```python
from build123d import *

# Parameters (mm, degrees)
SKETCH1_W           = 130
SKETCH1_H           = 120
BOSS_EXTRUDE1_DEPTH = 40
CUT_EXTRUDE1_DEPTH  = 40
CUT_EXTRUDE2_DEPTH  = 10
SKETCH4_R           = 10
CUT_EXTRUDE4_DEPTH  = 159
CUT_EXTRUDE5_DEPTH  = 20
SKETCH7_R           = 10
CUT_EXTRUDE6_DEPTH  = 20
CUT_EXTRUDE7_DEPTH  = 10


with BuildPart() as part:
    # Sketch1 → Boss-Extrude1 (new body)
    with BuildSketch(Plane.XY):
        with Locations((65, 60)):
            Rectangle(SKETCH1_W, SKETCH1_H)
    extrude(amount=BOSS_EXTRUDE1_DEPTH)

    # Sketch2 → Cut-Extrude1 (cut)
    with BuildSketch(Plane.XY.offset(40)):
        with BuildLine():
            Line((0, 70), (20, 70))
            ThreePointArc((20, 70), (30, 60), (20, 50))
            Line((20, 50), (0, 50))
            Line((0, 50), (0, 70))
        make_face()
    extrude(amount=-CUT_EXTRUDE1_DEPTH, mode=Mode.SUBTRACT)

    # Sketch3 → Cut-Extrude2 (cut)
    with BuildSketch(Plane.XY.offset(40)):
        with BuildLine():
            Line((20, 90), (0, 90))
            Line((0, 90), (0, 70))
            Line((0, 70), (20, 70))
            ThreePointArc((20, 70), (30, 60), (20, 50))
            Line((20, 50), (0, 50))
            Line((0, 50), (0, 30))
            Line((0, 30), (20, 30))
            ThreePointArc((20, 30), (50, 60), (20, 90))
        make_face()
    extrude(amount=-CUT_EXTRUDE2_DEPTH, mode=Mode.SUBTRACT)

    # Sketch4 → Cut-Extrude4 (cut)
    with BuildSketch(Plane.XY.offset(40)):
        with Locations((70, 60)):
            Circle(SKETCH4_R)
    extrude(amount=-CUT_EXTRUDE4_DEPTH, mode=Mode.SUBTRACT)

    # Sketch6 → Cut-Extrude5 (cut)
    with BuildSketch(Plane.XY.offset(30)):
        with BuildLine():
            Line((0, 90), (20, 90))
            ThreePointArc((20, 90), (50, 60), (20, 30))
            Line((20, 30), (0, 30))
            Line((0, 30), (0, 50))
            Line((0, 50), (20, 50))
            ThreePointArc((20, 50), (30, 60), (20, 70))
            Line((20, 70), (0, 70))
            Line((0, 70), (0, 90))
        make_face()
    extrude(amount=-CUT_EXTRUDE5_DEPTH, mode=Mode.SUBTRACT)

    # Sketch7 → Cut-Extrude6 (cut)
    with BuildSketch(Plane.XY.offset(40)):
        with BuildLine():
            Line((0, 120), (0, 90))
            Line((0, 90), (20, 90))
            ThreePointArc((20, 90), (50, 60), (20, 30))
            Line((20, 30), (0, 30))
            Line((0, 30), (0, 0))
            Line((0, 0), (70, 0))
            Line((70, 0), (70, 20))
            ThreePointArc((70, 20), (110, 60), (70, 100))
            Line((70, 100), (70, 120))
            Line((70, 120), (0, 120))
        make_face()
        with Locations((70, 60)):
            Circle(SKETCH7_R, mode=Mode.SUBTRACT)
    extrude(amount=-CUT_EXTRUDE6_DEPTH, mode=Mode.SUBTRACT)

    # Sketch8 → Cut-Extrude7 (cut)
    with BuildSketch(Plane.XY.offset(40)):
        with BuildLine():
            Line((96.457513111, 90), (130, 90))
            Line((130, 90), (130, 30))
            Line((130, 30), (96.457513111, 30))
            ThreePointArc((96.457513111, 30), (110, 60), (96.457513111, 90))
        make_face()
    extrude(amount=-CUT_EXTRUDE7_DEPTH, mode=Mode.SUBTRACT)


solid = part.part
```
Can you work these out from the model? Positions are in its coordinate system, mm. A direction names the side the tool comes from. Round coordinates to 2 decimals unless told otherwise and drop trailing zeros. Loops run counter-clockwise (first coordinate to the right, second up) from the corner with the lowest first, then second, coordinate; pieces in that order, holes last.
Item 1: Which directions (+Z, -Z, +X, -X, +Y, -Y) give clear straight access to the entire face, cutting with the end or side of a thin tool? Please do faces 1 (the flat face through (113, 90, 35)), 2 (the flat face through (70, 110, 30)), 3 (the flat face through (10, 30, 15)).
Item 2: Will these pins go through, and if not, where does the flat tip stop? pin 1 Ø6 at (y, z) = (14.5, 28) entering from -X; pin 2 Ø3 at (x, z) = (12, 17) entering from -Y; pin 3 Ø12 at (x, y) = (46.5, 18.5) entering from +Z; pin 4 Ø10 at (x, y) = (108.5, 50) entering from +Z.
Item 3: Suppose I cut it at C-C, the plane z = 4.5. Write out the boundary of the cut face in (x, y), then the cut area to 3 significant figures.
Item 4: If we mould it in two halves opening along X, with no side actions, what happens to faces 4 (the cylindrical face through (109.99, 59.12, 27.92)), 5 (the flat face through (54, 61, 20)), 6 (the cylindrical face through (60, 60, 10))? For each: +X half, -X half, draft (parallel to the pull), parting line (faces both ways), or undercut.
Item 5: Suppose I cut it at B-B, the plane y = 60. Write out the boundary of the cut face in (x, z).
Item 6: Suppose I cut it at D-D, the plane x = 81.5. Write out the boundary of the cut face in (y, z).
Item 7: Please list where these lines run through material, in increasing order: L1, parallel to Y at x = 70, z = 11; L2, parallel to Z at x = 21, y = 48; L3, parallel to X at y = 15, z = 24.5.
Item 8: Suppose I cut it at A-A, the plane z = 37.5. Write out the boundary of the cut face in (x, y).
Reported:
1. face 1: +Z, +X, -X
1. face 2: +Z, -X, +Y, -Y
1. face 3: +Z, -X
2. pin 1: stops at x = 70
2. pin 2: stops at y = 0
2. pin 3: stops at z = 20
2. pin 4: stops at z = 30
3. outline: (0, 0) - (130, 0) - (130, 120) - (0, 120) - (0, 70) - (20, 70) arc R10 cw to (20, 50) - (0, 50) - close; hole circle Ø20 at (70, 60)
3. area: 14,700 mm2
4. face 4: -X half
4. face 5: draft
4. face 6: undercut
5. outline: (30, 0) - (60, 0) - (60, 20) - (50, 20) - (50, 10) - (30, 10) - close; (80, 0) - (130, 0) - (130, 30) - (110, 30) - (110, 20) - (80, 20) - close
6. outline: (0, 0) - (120, 0) - (120, 40) - (98.31, 40) - (98.31, 20) - (21.69, 20) - (21.69, 40) - (0, 40) - close
7. L1: y = 0 to 50, 70 to 120
7. L2: z = 0 to 10
7. L3: x = 70 to 130
8. outline: (70, 0) - (130, 0) - (130, 30) - (96.46, 30) arc R40 cw to (70, 20) - close; (70, 100) arc R40 cw to (96.46, 90) - (130, 90) - (130, 120) - (70, 120) - close
